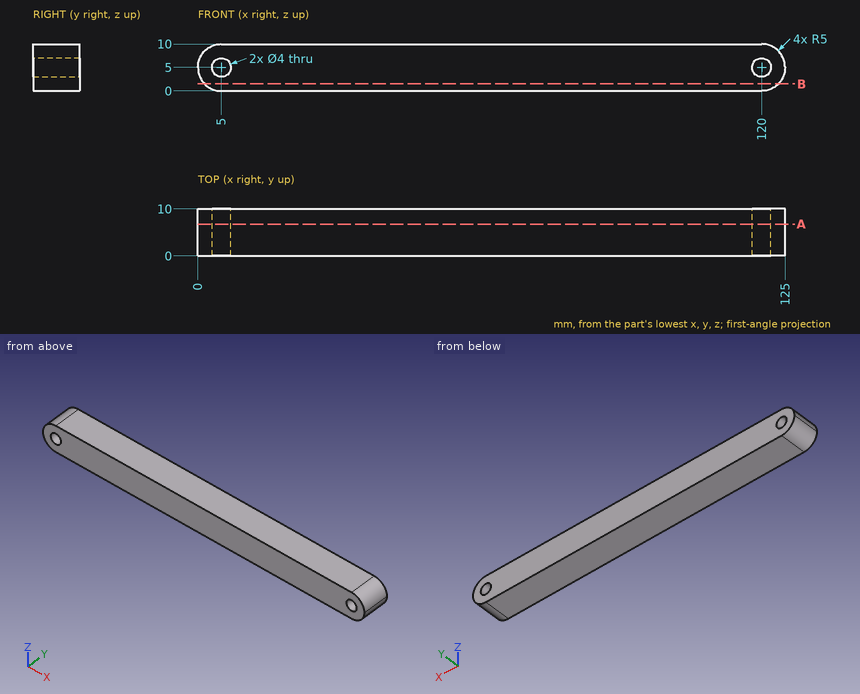
Study the drawing (mm; zero at the part's minimum x, y, z) and answer. Give positions to 0.01 mm unless a question says otherwise; leave off trailing zeros. Write each loop counter-clockwise with the first axis right and the second up, starting at its lowest first coordinate (ties: lowest second). Pieces come first, ordered by that corner, then holes. Notation, with made-up numbers: (-38.75, 32.25) - (-13.75, 32.25) arc R16 cw to (-13.75, 41.25) - close; hole circle Ø7 at (30.5, -40). An arc over 180 degrees is marked (long way). Use a Markdown table: item, result.
1. Each of these flat-tipped pins is pushed along its axis until it touches: P1, Ø1, axis at y = 8.5, z = 2.5, coming from the -X side; P2, Ø1.5, axis at y = 2, z = 3, coming from the -X side. Where does it stop, or does it pass through?
Values follow:
| item | result |
|---|---|
| P1 | stops at x = 0.42 |
| P2 | stops at x = 0.16 |
2. Section A-A on y = 6.75 is taken. Count the separate pieces of the cut face and the enclosed holes in it, plus the area to 3 significant figures.
Values follow:
| item | result |
|---|---|
| separate pieces | 1 |
| enclosed holes | 2 |
| area | 1,200 mm² |
3. Find the intervals of material crossed by probe 1 along X at (y, z) = (2, 5); probe 2 along Z at (x, y) = (120, 5.5); probe 3 along X at (y, z) = (5.5, 4.5) (1 decimal), in increasing order. Write a range as from..to.
Values follow:
| item | result |
|---|---|
| probe 1 | x = 0..3, 7..118, 122..125 |
| probe 2 | z = 0..3, 7..10 |
| probe 3 | x = 0..3.1, 6.9..118.1, 121.9..125 |
4. Section B-B on z = 1.5 is taken. Write down the section's boundary in (x, y).
Values follow:
| item | result |
|---|---|
| outline | (1.43, 0) - (123.57, 0) - (123.57, 10) - (1.43, 10) - close |
